from build123d import *

# Parameters (mm, degrees)
SKETCH1_R                      = 70
BOSS_EXTRUDE2_DEPTH            = 12.7
FILLET1_R                      = 1
CHAMFER1_SIZE                  = 2.232593028
CHAMFER1_SIZE_2                = 2.5
F_3_0MM_DOWEL_HOLE2_REACH      = 215.907
F_3_0MM_DOWEL_HOLE2_BORE_R     = 1.65
CIRPATTERN3_COUNT              = 3
SKETCH8_W                      = 2
SKETCH8_H                      = 7.5
CUT_EXTRUDE1_DEPTH             = 142.990457435
FILLET2_R                      = 0.25
CIRPATTERN4_COUNT              = 3
FILLET2_OF_CIRPATTERN4_R       = 0.25
CBORE_FOR_M3_SHCS1_D           = 3.4
CBORE_FOR_M3_SHCS1_DEPTH       = 25.25
CBORE_FOR_M3_SHCS1_CBORE_D     = 6.5
CBORE_FOR_M3_SHCS1_CBORE_DEPTH = 3
CBORE_FOR_M3_SHCS1_TIP         = 1.021463052
F_3_0MM_DOWEL_HOLE3_D          = 3.3
F_3_0MM_DOWEL_HOLE3_DEPTH      = 45
F_3_0MM_DOWEL_HOLE3_TIP        = 0.991420021


with BuildPart() as part:
    # Sketch1 → Boss-Extrude2 (new body)
    with BuildSketch(Plane(origin=(0, 0, 0), x_dir=(1, 0, 0), z_dir=(0, 1, 0))):
        with BuildLine():
            ThreePointArc((100, 0), (89.630863423, 44.343075243), (60.673833561, 79.490162417))
            Line((60.673833561, 79.490162417), (48.335125168, 58.118892582))
            Line((48.335125168, 58.118892582), (26.164874832, 70.918892582))
            Line((26.164874832, 70.918892582), (38.503583224, 92.290162417))
            ThreePointArc((38.503583224, 92.290162417), (-50, 86.602540378), (-99.177416784, 12.8))
            Line((-99.177416784, 12.8), (-74.5, 12.8))
            Line((-74.5, 12.8), (-74.5, -12.8))
            Line((-74.5, -12.8), (-99.177416784, -12.8))
            ThreePointArc((-99.177416784, -12.8), (-50, -86.602540378), (38.503583224, -92.290162417))
            Line((38.503583224, -92.290162417), (26.164874832, -70.918892582))
            Line((26.164874832, -70.918892582), (48.335125168, -58.118892582))
            Line((48.335125168, -58.118892582), (60.673833561, -79.490162417))
            ThreePointArc((60.673833561, -79.490162417), (89.630863423, -44.343075243), (100, 0))
        make_face()
        with Locations(Location((0, 0, 0), (0, 0, 270))):
            Circle(SKETCH1_R, mode=Mode.SUBTRACT)
    extrude(amount=BOSS_EXTRUDE2_DEPTH)

    # Fillet1
    fillet1_edges = [part.edges().sort_by_distance(p)[0] for p in [
        (48.335125168, 6.35, 58.118892582),
        (26.164874832, 6.35, 70.918892582),
        (-74.5, 6.35, 12.8),
        (-74.5, 6.35, -12.8),
        (26.164874832, 6.35, -70.918892582),
        (48.335125168, 6.35, -58.118892582),
    ]]
    fillet(fillet1_edges, radius=FILLET1_R)

    # Chamfer1
    # the kernel refuses this chamfer: 2.5, 2.232593028 mm, written as the material it takes off along each edge
    with BuildSketch(Plane(origin=(38.503583224, -6.351330223, 92.290162417), x_dir=(-0.4999999999994457, 0, -0.8660254037847587), z_dir=(0, 1, 0)), Plane(origin=(60.673833561, -6.351330223, -79.490162417), x_dir=(-0.5000000000003051, 0, 0.8660254037842624), z_dir=(0, 1, 0))) as chamfer1_piece_1:
        with BuildLine():
            Line((CHAMFER1_SIZE, 0), (0.346342416, 2.445285803))
            ThreePointArc((0.346342416, 2.445285803), (0.170523224, 1.258272567), (0, 0))
            Line((0, 0), (CHAMFER1_SIZE, 0))
        make_face()
    extrude(amount=25.402660447, mode=Mode.SUBTRACT)
    with BuildSketch(Plane(origin=(-99.177416784, -6.42920747, 12.8), x_dir=(0.13897023449143497, 0, 0.990296558574953), z_dir=(0, 1, 0)), Plane(origin=(60.673833561, -6.42920747, 79.490162417), x_dir=(0.7881368597604604, 0, -0.6155000327269856), z_dir=(0, 1, 0))) as chamfer1_piece_2:
        with BuildLine():
            Line((2.213825834, 0), (CHAMFER1_SIZE_2 * 0.138970234491, CHAMFER1_SIZE_2 * 0.990296558575))
            Line((CHAMFER1_SIZE_2 * 0.138970234491, CHAMFER1_SIZE_2 * 0.990296558575), (0, 0))
            ThreePointArc((0, 0), (1.137001677, -0.006121942), (2.213825834, 0))
        make_face()
    extrude(amount=25.55841494, mode=Mode.SUBTRACT)
    with BuildSketch(Plane(origin=(-99.177416784, -6.351330223, -12.8), x_dir=(0.1402371214073107, 0, -0.9901179474079799), z_dir=(0, 1, 0))) as chamfer1_piece_3:
        with BuildLine():
            Line((2.469691423, 0), (CHAMFER1_SIZE * 0.140237121404, -CHAMFER1_SIZE * 0.990117947384))
            Line((CHAMFER1_SIZE * 0.140237121404, -CHAMFER1_SIZE * 0.990117947384), (0, 0))
            ThreePointArc((0, 0), (1.269751938, 0.007618418), (2.469691423, 0))
        make_face()
    extrude(amount=25.402660447, mode=Mode.SUBTRACT)
    with BuildSketch(Plane(origin=(38.503583224, -6.42920747, -92.290162417), x_dir=(-0.49999999999948913, 0, 0.8660254037847336), z_dir=(0, 1, 0))) as chamfer1_piece_4:
        with BuildLine():
            Line((CHAMFER1_SIZE_2, 0), (0.307655895, -2.192344105))
            ThreePointArc((0.307655895, -2.192344105), (0.151946852, -1.126819615), (0, 0))
            Line((0, 0), (CHAMFER1_SIZE_2, 0))
        make_face()
    extrude(amount=25.55841494, mode=Mode.SUBTRACT)

    # Ø3.0mm Dowel Hole2 bore → Ø3.0mm Dowel Hole2 (cut, up to next)
    with BuildSketch(Plane(origin=(37.25, 0, 64.518892582), x_dir=(0.8660254037844382, 0, -0.500000000000001), z_dir=(0.5000000000000009, 0, 0.866025403784438)), mode=Mode.PRIVATE) as f_3_0mm_dowel_hole2_sk1:
        with Locations((0, 6.35)):
            Circle(F_3_0MM_DOWEL_HOLE2_BORE_R)
    f_3_0mm_dowel_hole2_tool1 = extrude(f_3_0mm_dowel_hole2_sk1.sketch, amount=-F_3_0MM_DOWEL_HOLE2_REACH, mode=Mode.PRIVATE) & part.part
    f_3_0mm_dowel_hole2 = f_3_0mm_dowel_hole2_tool1.solids().sort_by_distance((37.25, 6.35, 64.518893))[0]
    add(f_3_0mm_dowel_hole2, mode=Mode.SUBTRACT)

    # CirPattern3: Ø3.0mm Dowel Hole2 ×3 about axis
    cirpattern3_axis = Axis((0, 12.7, 0), (0, -1, 0))
    for i in range(1, CIRPATTERN3_COUNT):
        add(f_3_0mm_dowel_hole2.rotate(cirpattern3_axis, i * 360 / CIRPATTERN3_COUNT), mode=Mode.SUBTRACT)

    # Sketch8 → Cut-Extrude1 (cut, through all)
    with BuildSketch(Plane(origin=(0, 12.7, 0), x_dir=(1, 0, 0), z_dir=(0, 1, 0))):
        with Locations((-70, 0)):
            Rectangle(SKETCH8_W, SKETCH8_H)
    cut_extrude1 = extrude(amount=-CUT_EXTRUDE1_DEPTH, mode=Mode.SUBTRACT)

    # Fillet2
    fillet2_edges = [part.edges().sort_by_distance(p)[0] for p in [
        (-69.8994814, 6.35, 3.75),
        (-69.8994814, 6.35, -3.75),
        (-71, 6.35, 3.75),
        (-71, 6.35, -3.75),
    ]]
    fillet(fillet2_edges, radius=FILLET2_R)

    # CirPattern4: Cut-Extrude1 ×3 about axis
    cirpattern4_axis = Axis((0, 0, 0), (0, 1, 0))
    for i in range(1, CIRPATTERN4_COUNT):
        add(cut_extrude1.rotate(cirpattern4_axis, i * 360 / CIRPATTERN4_COUNT), mode=Mode.SUBTRACT)

    # Fillet2 of CirPattern4
    fillet2_of_cirpattern4_edges = [part.edges().sort_by_distance(p)[0] for p in [
        (38.197335964, 6.35, 58.659726604),
        (31.702145436, 6.35, 62.409726604),
        (38.747595264, 6.35, 59.612803669),
        (32.252404736, 6.35, 63.362803669),
        (31.702145436, 6.35, -62.409726604),
        (38.197335964, 6.35, -58.659726604),
        (32.252404736, 6.35, -63.362803669),
        (38.747595264, 6.35, -59.612803669),
    ]]
    fillet(fillet2_of_cirpattern4_edges, radius=FILLET2_OF_CIRPATTERN4_R)

    # CBORE for M3 SHCS1
    with Locations(Plane(origin=(0, 12.7, 0), x_dir=(1, 0, 0), z_dir=(0, 1, 0))):
        with Locations((6, 88.602076866), (-6, 88.602076866)):
            CounterBoreHole(CBORE_FOR_M3_SHCS1_D / 2, CBORE_FOR_M3_SHCS1_CBORE_D / 2, CBORE_FOR_M3_SHCS1_CBORE_DEPTH, depth=CBORE_FOR_M3_SHCS1_DEPTH)
            with Locations((0, 0, -(CBORE_FOR_M3_SHCS1_DEPTH + CBORE_FOR_M3_SHCS1_TIP / 2))):  # 118° drill point
                Cone(0, CBORE_FOR_M3_SHCS1_D / 2, CBORE_FOR_M3_SHCS1_TIP, mode=Mode.SUBTRACT)

    # Ø3.0mm Dowel Hole3
    with Locations(Plane(origin=(0, 12.7, 0), x_dir=(1, 0, 0), z_dir=(0, 1, 0))):
        with Locations((12, -79.094879733), (12, -89.196412484), (-12, -89.196412484), (-12, -79.094879733)):
            Hole(F_3_0MM_DOWEL_HOLE3_D / 2, depth=F_3_0MM_DOWEL_HOLE3_DEPTH)
            with Locations((0, 0, -(F_3_0MM_DOWEL_HOLE3_DEPTH + F_3_0MM_DOWEL_HOLE3_TIP / 2))):  # 118° drill point
                Cone(0, F_3_0MM_DOWEL_HOLE3_D / 2, F_3_0MM_DOWEL_HOLE3_TIP, mode=Mode.SUBTRACT)


solid = part.part
The listing builds one solid part. Answer for the finished solid, in the listing's coordinates (mm). A direction names the side the tool comes from. Give positions to 0.01 mm unless a question says otherwise; leave off trailing zeros. Order: outer loops, then holes, each group sorted by start corner. A loop starts at its lowest first (then second) coordinate and runs counter-clockwise, first axis right, second up. Notation, with made-up numbers: (71.5, 50.25) - (78.5, 50.25) arc R23 ccw to (78.5, 88.25) - close; hole circle Ø6 at (46, 32). An arc over 180 degrees is marked (long way). One line per item, written item: value. Start each with the question number.
1) A tool of negligible diameter and unlimited length cuts with its end or side. For faces 1 (the face through (69.993, 6.261, 0.97)), 2 (the face through (-6.7, 11.22, -85.43)), 3 (the face through (-51.2, 6.3, 85.9)), 4 (the face through (54.27, 6.26, -68.4)), from which of +Z, -Z, +X, -X, +Y, -Y can it reach the whole face along a straight path? Write none if from no direction.
2) Given pin 1 Ø2 at (x, z) = (12, 79.09) entering from -Y; pin 2 Ø0.7 at (x, y) = (-70.5, 3) entering from +Z; pin 3 Ø1.5 at (x, y) = (-65.5, 11) entering from -Z; pin 4 Ø6 at (x, y) = (-4.5, 9) entering from -Z, each flat-ended and moving along its own axis, determine where each tip first touches the part or whether it passes through.
3) The mould has two halves that part along X. Classify faces 5 (the face through (-86, 6, 12.8)), 6 (the face through (-5, 9.7, -87)), 7 (the face through (-74.5, 6, -3)), 8 (the face through (34.84, 6.26, 65.91)): released by +X, released by -X, zero draft, split by the parting line, or undercut.
4) A cutting plane is placed at A-A on z = 41.5. Give the vertices of the cut face in (x, y), then the cut area to 3 significant figures.
5) Find the intervals of material crossed by L1, parallel to Z at x = -6, y = 3.5; L2, parallel to Z at x = -12, y = 6.5; L3, parallel to Z at x = 13, y = 5, in increasing order.
6) A cutting plane is placed at B-B on x = -78.5. Give the vertices of the cut face in (y, z), then the cut area to 3 significant figures.
Answer sheet:
1. face 1: +Y, -Y
1. face 2: +Y
1. face 3: +Z, +Y, -Y
1. face 4: -Z, +Y, -Y
2. pin 1: passes through
2. pin 2: stops at z = 71.27
2. pin 3: stops at z = -76.21
2. pin 4: stops at z = -99.99
3. face 5: zero draft
3. face 6: undercut
3. face 7: released by -X
3. face 8: undercut
4. outline: (-90.98, 0) - (-56.37, 0) - (-56.37, 12.7) - (-90.98, 12.7) - close; (56.37, 0) - (90.98, 0) - (90.98, 12.7) - (56.37, 12.7) - close
4. area: 879 mm2
5. L1: z = -99.82 to -90.3, -86.9 to -69.74, 69.74 to 99.82
5. L2: z = -99.28 to -68.96, 68.96 to 77.44, 80.74 to 87.55, 90.85 to 99.28
5. L3: z = -99.15 to -68.78, 68.78 to 77.78, 80.41 to 87.88, 90.51 to 99.15
6. outline: (0, -61.95) - (12.7, -61.95) - (12.7, -12.8) - (0, -12.8) - close; (0, 12.8) - (12.7, 12.8) - (12.7, 61.95) - (0, 61.95) - close
6. area: 1,250 mm2
